Build history of the part. All positions in model axes, mm. A direction names the side the tool comes from. Round coordinates to 2 decimals unless told otherwise and drop trailing zeros. Loops run counter-clockwise (first coordinate to the right, second up) from the corner with the lowest first, then second, coordinate; pieces in that order, holes last. Notation, with made-up numbers: (13.25, -21.75) - (41.25, -21.75) arc R16 cw to (41.25, 5.25) - close; hole circle Ø11 at (25, 84.25). An arc over 180 degrees is marked (long way). Use a Markdown table: item, result.
from build123d import *

# Parameters (mm, degrees)
F3_START = 10
F2_W     = 1.5
F2_H     = 19
F2_W_2   = 19
F2_H_2   = 1.5
F3_DEPTH = 15


with BuildPart() as f1:
    # F0 (on Front) → F1 (revolve)
    with BuildSketch(Plane.XZ):
        with BuildLine():
            ThreePointArc((-2, 28.5), (-1.4142135624, 27.0857864376), (0, 26.5))
            Line((0, 26.5), (25, 26.5))
            Line((25, 26.5), (25, 27.5))
            Line((25, 27.5), (0, 27.5))
            ThreePointArc((0, 27.5), (-0.7071067812, 27.7928932188), (-1, 28.5))
            Line((-1, 28.5), (-2, 28.5))
        make_face()
    revolve(axis=Axis((19.6649903227, 0, 0), (1, 0, 0)))



with BuildPart() as f1b:
    # F0 (on Front) → F1, piece 2 (revolve)
    with BuildSketch(Plane.XZ):
        with BuildLine():
            Line((0, 1), (0, 0))
            Line((0, 0), (36.5830052443, 0))
            Line((36.5830052443, 0), (36.5830052443, 9))
            Line((36.5830052443, 9), (10.5830052443, 9))
            ThreePointArc((10.5830052443, 9), (3.9497556635, 6.7749643874), (0, 1))
        make_face()
    revolve(axis=Axis((19.6649903227, 0, 0), (1, 0, 0)))


with BuildPart() as f1_1:
    add(f1.part)

    add(f1b.part)  # F3 merges F1b
    # F2 (on Right) → F3 (join)
    with BuildSketch(Plane.YZ.offset(F3_START)):
        with Locations((0, 17.5)):
            Rectangle(F2_W, F2_H)
        with Locations((-17.5, 0)):
            Rectangle(F2_W_2, F2_H_2)
        with Locations((0, -17.5)):
            Rectangle(F2_W, F2_H)
        with Locations((17.5, 0)):
            Rectangle(F2_W_2, F2_H_2)
    extrude(amount=F3_DEPTH)


solid = f1_1.part
Q1. Cut at D-D, the plane x = 27.5. List the corners of the cut face in (y, z), plus the area to 3 significant figures.
Results found:
| item | result |
|---|---|
| outline | circle Ø18 at (0, 0) |
| area | 254 mm2 |
Q2. Cut at B-B, the plane z = -8. Count the separate pieces of the cut face and the enclosed holes in it, plus the area to 3 significant figures.
Results found:
| item | result |
|---|---|
| separate pieces | 3 |
| enclosed holes | 0 |
| area | 301 mm2 |
Q3. Pull direction Y, two halves, no side cores. Call faces 4 (the face through (36.583, 0, 0)), 5 (the face through (12.325, 26.846, -5.961)), 6 (the face through (10, -18, 0)), 7 (the face through (10, 0, 18)): pulls with the +Y half, pulls with the -Y half, needs draft (parallel to the pull), parting line crosses it, or undercut.
Results found:
| item | result |
|---|---|
| face 4 | needs draft |
| face 5 | parting line crosses it |
| face 6 | undercut |
| face 7 | undercut |
Q4. Cut at A-A, the plane x = 14. List the corners of the cut face in (y, z), plus the area to 3 significant figures.
Results found:
| item | result |
|---|---|
| outline | circle Ø55 at (0, 0); hole (-26.49, -0.75) arc R26.5 ccw to (-0.75, -26.49) - (-0.75, -8.97) arc R9 cw to (-8.97, -0.75) - close; hole (-26.49, 0.75) - (-8.97, 0.75) arc R9 cw to (-0.75, 8.97) - (-0.75, 26.49) arc R26.5 ccw to start; hole (0.75, -26.49) arc R26.5 ccw to (26.49, -0.75) - (8.97, -0.75) arc R9 cw to (0.75, -8.97) - close; hole (0.75, 8.97) arc R9 cw to (8.97, 0.75) - (26.49, 0.75) arc R26.5 ccw to (0.75, 26.49) - close |
| area | 529 mm2 |
Q5. Probe line 1 (Y direction, x = 11, z = 14); line 2 (Y direction, x = 6.5, z = 0); line 3 (Z direction, x = 10.5, y = 10). List the from-to ranges inside material, lowest first.
Results found:
| item | result |
|---|---|
| line 1 | y = -23.67 to -22.5, -0.75 to 0.75, 22.5 to 23.67 |
| line 2 | y = -27.5 to -26.5, -8.21 to 8.21, 26.5 to 27.5 |
| line 3 | z = -25.62 to -24.54, -0.75 to 0.75, 24.54 to 25.62 |
Q6. Drop flat-ended pins along their axis: pin 1 (2 mm diameter, centred on x = 22, z = -16.5, fed in from +Y); pin 2 (12 mm diameter, centred on x = 14.5, y = 21.5, fed in from +Z); pin 3 (7.5 mm diameter, centred on x = 16, y = 19.5, fed in from -Z); pin 4 (5 mm diameter, centred on y = -19, z = -3.5, fed in from -X). Give the stop position or say it passes through.
Results found:
| item | result |
|---|---|
| pin 1 | stops at y = 22.72 |
| pin 2 | stops at z = 22.72 |
| pin 3 | stops at z = -22.54 |
| pin 4 | passes through |
Q7. Which spindle directions (+Z, -Z, +X, -X, +Y, -Y) get a long thin tool onto all of the face, cutting with end or side? Do faces 1 (the face through (25, -10, 0)), 2 (the face through (10, 18, 0)), 3 (the face through (17, 0.75, 18)). Say none if no direction does.
Results found:
| item | result |
|---|---|
| face 1 | +X |
| face 2 | -X |
| face 3 | +X, -X |
